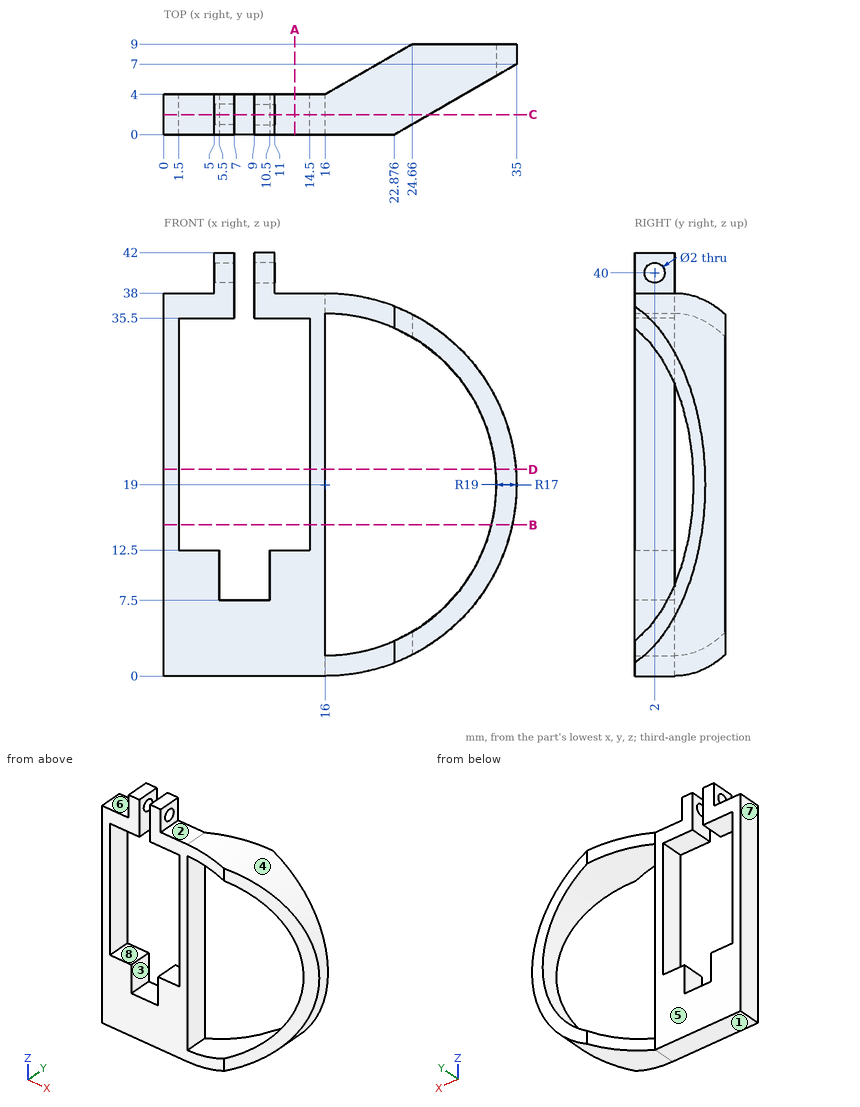
Study the drawing (mm; zero at the part's minimum x, y, z) and answer. A direction names the side the tool comes from. Round coordinates to 2 decimals unless told otherwise and drop trailing zeros. Write each loop counter-clockwise with the first axis right and the second up, starting at its lowest first coordinate (ties: lowest second). Pieces come first, ordered by that corner, then holes. Notation, with made-up numbers: (22, -9) - (41, -9) arc R19 ccw to (41, 14) - close; hole circle Ø6 at (-26.5, 52.25). An arc over 180 degrees is marked (long way). Use CSV: the item, a comma, the result in double quotes.
Q1. Straight lines are drawn through the part: line 1 along Z through (x, y) = (13.5, 2.5); line 2 along Y through (x, z) = (9.65, 40); line 3 along X through (y, z) = (1.5, 16.5). For each, find the intervals that lie inside material, in ascending order.
Values:
line 1,"z = 0 to 12.5, 35.5 to 38"
line 2,"y = 0 to 1, 3 to 4"
line 3,"x = 0 to 1.5, 14.5 to 16"
Q2. Determine the mould class of the marked faces 1, 2 and 3 for opening direction Z: +Z half, -Z half, draft (parallel to the pull), parting line (faces both ways), or undercut.
Values:
face 1,"-Z half"
face 2,"+Z half"
face 3,"undercut"
Q3. A tool of negligible diameter and unlimited length cuts with its end or side. For the marked faces 4, 5, 6, 7 and 8, from which of +Z, -Z, +X, -X, +Y, -Y can it reach the whole face along a straight path? Write none if from no direction.
Values:
face 4,"+X, +Y, -Y"
face 5,"+Z, -Z, -X, +Y"
face 6,"+Z, -X, +Y, -Y"
face 7,"+Z, -Z, -X, +Y, -Y"
face 8,"+Y, -Y"
Q4. Find section B-B, the plane z = 15. Write down the section's boundary in (x, y).
Values:
outline,"(0, 0) - (1.5, 0) - (1.5, 4) - (0, 4) - close; (14.5, 0) - (16, 0) - (16, 4) - (14.5, 4) - close; (32.52, 5.57) - (34.57, 6.75) - (34.57, 9) - (32.52, 9) - close"
Q5. Find section D-D, the plane z = 20.5. Write down the section's boundary in (x, y).
Values:
outline,"(0, 0) - (1.5, 0) - (1.5, 4) - (0, 4) - close; (14.5, 0) - (16, 0) - (16, 4) - (14.5, 4) - close; (32.93, 5.81) - (34.94, 6.97) - (34.94, 9) - (32.93, 9) - close"
Q6. Find section A-A, the plane x = 13. Write down the section's boundary in (y, z), then the cut area to 3 significant figures.
Values:
outline,"(0, 0) - (4, 0) - (4, 12.5) - (0, 12.5) - close; (0, 35.5) - (4, 35.5) - (4, 38) - (0, 38) - close"
area,"60.0 mm²"
Q7. Find section C-C, the plane y = 2. Count the separate pieces of the cut face and the enclosed holes in it, then the cut area to 3 significant figures.
Values:
separate pieces,"3"
enclosed holes,"0"
area,"331 mm²"
Q8. Each of these flat-tipped pins is pushed along its axis until it touches: pin 1 Ø2 at (y, z) = (1.5, 27) entering from -X; pin 2 Ø1.2 at (x, y) = (14, 2) entering from +Z; pin 3 Ø2 at (y, z) = (3, 41) entering from -X; pin 4 Ø4.5 at (y, z) = (2.5, 20.5) entering from +X. Where does it stop, or does it pass through?
Values:
pin 1,"stops at x = 0"
pin 2,"stops at z = 38"
pin 3,"stops at x = 5"
pin 4,"stops at x = 16"
